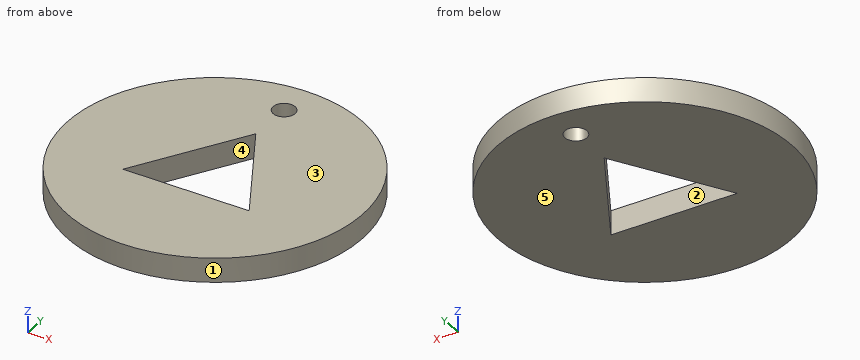
```python
from build123d import *

# Parameters (mm, degrees)
CYLINDER_R      = 20
CYLINDER_DEPTH  = 3.3
SKETCH_R        = 1.5
POCKET_DEPTH    = 3.301
POCKET001_DEPTH = 3.301


with BuildPart() as part:
    # Cylinder → Cylinder (new body)
    with BuildSketch(Plane.XY):
        Circle(CYLINDER_R)
    extrude(amount=CYLINDER_DEPTH)

    # Sketch → Pocket (cut, through all)
    with BuildSketch(Plane.XY.offset(3.3)):
        with Locations((0, 15.1)):
            Circle(SKETCH_R)
    extrude(amount=-POCKET_DEPTH, mode=Mode.SUBTRACT)

    # Sketch001 → Pocket001 (cut, through all)
    with BuildSketch(Plane.XY.offset(3.3)):
        Polygon((0, 8.915402), (-8.923643, -5.938961), (8.405048, -5.938961), align=None)
    extrude(amount=-POCKET001_DEPTH, mode=Mode.SUBTRACT)


solid = part.part
```
Can you work these out from the model? Positions are in its coordinate system, mm. Face numbers are marked on the shaded views. A direction names the side the tool comes from. Round coordinates to 2 decimals unless told otherwise and drop trailing zeros. Order: outer loops, then holes, each group sorted by start corner. A loop starts at its lowest first (then second) coordinate and runs counter-clockwise, first axis right, second up. Notation, with made-up numbers: (9, 71) -> (22, 71) arc R32 cw to (22, 101) -> close; hole circle Ø1 at (-8.75, 35). An arc over 180 degrees is marked (long way). Return JSON: item names as keys, results as strings. Group by question number.
1. Will these pins go through, and if not, where does the flat tip stop? pin 1 (1 mm diameter, centred on x = 11, z = 3, fed in from -Y); pin 2 (1.5 mm diameter, centred on y = 10.5, z = 2, fed in from +X).
2. Which directions (+Z, -Z, +X, -X, +Y, -Y) give clear straight access to the entire face, cutting with the end or side of a thin tool? Please do the marked faces 4 and 5.
3. We'd pull the mould along X, two halves only. Please class the marked faces 1, 2 and 3: released by +X, released by -X, zero draft, split by the parting line, or undercut.
4. I need wall thicknesses on line 1 (Y direction, x = -7, z = 2.3) (3 decimals); line 2 (X direction, y = -4, z = 2); line 3 (X direction, y = -3.5, z = 3). Which ranges of each line are inside material? Lowest first, please. Write a range as [from, to].
5. If we section it at D-D, the plane x = 16: Write out the boundary of the cut face in (y, z).
6. If we section it at C-C, the plane y = 15.1: Write out the boundary of the cut face in (x, z), then the cut area to 3 significant figures.
7. If we section it at B-B, the plane x = -8: Write out the boundary of the cut face in (y, z), then the cut area to 3 significant figures.
8. If we section it at A-A, the plane z = 0.6: Write out the boundary of the cut face in (x, y).
Output values:
{
 "1": {"pin 1": "y = -17.02", "pin 2": "x = 17.46"},
 "2": {"face 4": "+Z, -Z", "face 5": "-Z, +X, -X, +Y, -Y"},
 "3": {"face 1": "split by the parting line", "face 2": "undercut", "face 3": "zero draft"},
 "4": {"line 1": "[-18.735, -5.939], [-2.737, 18.735]", "line 2": "[-19.6, -7.76], [7.31, 19.6]", "line 3": "[-19.69, -7.46], [7.03, 19.69]"},
 "5": {"outline": "(-12, 0) -> (12, 0) -> (12, 3.3) -> (-12, 3.3) -> close"},
 "6": {"outline": "(-13.11, 0) -> (-1.5, 0) -> (-1.5, 3.3) -> (-13.11, 3.3) -> close; (1.5, 0) -> (13.11, 0) -> (13.11, 3.3) -> (1.5, 3.3) -> close", "area": "76.7 mm²"},
 "7": {"outline": "(-18.33, 0) -> (-5.94, 0) -> (-5.94, 3.3) -> (-18.33, 3.3) -> close; (-4.4, 0) -> (18.33, 0) -> (18.33, 3.3) -> (-4.4, 3.3) -> close", "area": "116 mm²"},
 "8": {"outline": "circle Ø40 at (0, 0); hole (-8.92, -5.94) -> (8.41, -5.94) -> (0, 8.92) -> close; hole circle Ø3 at (0, 15.1)"}
}
